Source: CAD feature listing. Evaluate the final solid. Frame: model axes, mm. Face numbers are marked on the shaded views. A direction names the side the tool comes from. Give positions to 0.01 mm unless a question says otherwise; leave off trailing zeros. Write each loop counter-clockwise with the first axis right and the second up, starting at its lowest first coordinate (ties: lowest second). Pieces come first, ordered by that corner, then holes. Notation, with made-up numbers: M 61.25,45 L 109.25,45 A20 ccw 109.25,71 Z; hole C 14,85.25 d7. An arc over 180 degrees is marked long. Use CSV: the item, a comma, the result in double quotes. Start each with the question number.
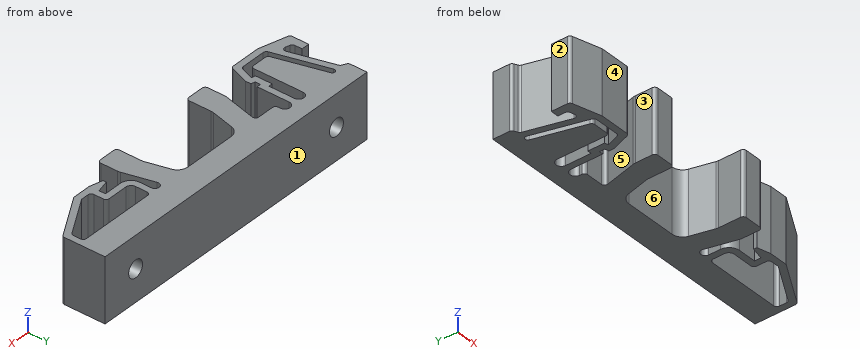
from build123d import *

# Parameters (mm, degrees)
BOSS_EXTRUDE1_DEPTH     = 6
CUT_EXTRUDE1_DEPTH      = 35.525353003
CUT_EXTRUDE1_DEPTH_BACK = 35.525353003
FILLET1_R               = 2
FILLET2_R               = 1
FILLET3_R               = 0.811424
FILLET4_R               = 2
FILLET5_R               = 1
FILLET6_R               = 1
FILLET7_R               = 0.5
FILLET8_R               = 0.6
SKETCH4_R               = 1.6
CUT_EXTRUDE2_DEPTH      = 8.5


with BuildPart() as part:
    # Sketch2 → Boss-Extrude1 (new, symmetric)
    with BuildSketch(Plane.XY):
        Polygon((6.5, 11), (-6.5, 11), (-8, 4.9838286), (-8, 0), (-12.25, 0), (-12.25, 3.981133366), (-10.5, 11), (-15, 11), (-15, 13), (-17, 13), (-17, 6), (-17.75, 6), (-17.75, 5), (-17, 4.813003998), (-17, 3.813003998), (-18.387819958, 0), (-24.387819958, 0), (-30, 1.50377911), (-30, 5.00377911), (-28.5, 5.00377911), (-28.5, 3.172407682), (-26.2783706, 2.577123878), (-28.785442178, 11.933642386), (-30, 12.5), (-30, 16), (0, 16), (30, 16), (30, 8), (21.339745962, 3), (17.839745962, 3), (15.4, 3.608296988), (15.4, 4.214079193), (17.75, 4.8), (17.75, 6), (12.35, 6), (12.35, 11), (10.5, 11), (12.25, 3.981133366), (12.25, 0), (8, 0), (8, 4.9838286), align=None)
    extrude(amount=BOSS_EXTRUDE1_DEPTH, both=True)

    # Sketch3 → Cut-Extrude1 (cut, two sides: drawn at the far end of the back side and taken through both)
    with BuildSketch(Plane.XY.offset(-CUT_EXTRUDE1_DEPTH_BACK)):
        Polygon((-27.626331186, 12.24422524), (-24.667039952, 1.2), (-19.228069004, 1.2), (-18.249764702, 3.88786898), (-18.95, 4.062457248), (-18.95, 7.2), (-18.2, 7.2), (-18.2, 13), (-20.2, 13), (-20.2, 2.2), (-23.899712964, 2.2), (-26.66040536, 12.503044285), align=None)
        Polygon((13.55, 11), (13.55, 7.2), (18.95, 7.2), (18.95, 4.2), (21.018206931, 4.2), (28.8, 8.692820323), (28.8, 11), align=None)
    extrude(amount=CUT_EXTRUDE1_DEPTH + CUT_EXTRUDE1_DEPTH_BACK, mode=Mode.SUBTRACT)

    # Fillet1
    fillet1_edges = [part.edges().sort_by_distance(p)[0] for p in [
        (12.35, 6, 0),
    ]]
    fillet(fillet1_edges, radius=FILLET1_R)

    # Fillet2
    fillet2_edges = [part.edges().sort_by_distance(p)[0] for p in [
        (13.55, 7.2, 0),
    ]]
    fillet(fillet2_edges, radius=FILLET2_R)

    # Fillet3
    fillet3_edges = [part.edges().sort_by_distance(p)[0] for p in [
        (12.35, 11, 0),
        (10.5, 11, 0),
    ]]
    fillet(fillet3_edges, radius=FILLET3_R)

    # Fillet4
    fillet4_edges = [part.edges().sort_by_distance(p)[0] for p in [
        (12.25, 3.981133366, 0),
        (8, 4.9838286, 0),
        (6.5, 11, 0),
        (-6.5, 11, 0),
        (-8, 4.9838286, 0),
        (-12.25, 3.981133366, 0),
    ]]
    fillet(fillet4_edges, radius=FILLET4_R)

    # Fillet5
    fillet5_edges = [part.edges().sort_by_distance(p)[0] for p in [
        (-20.2, 13, 0),
        (-18.2, 13, 0),
    ]]
    fillet(fillet5_edges, radius=FILLET5_R - 0.0001)  # a hair under: the kernel refuses the full size

    # Fillet6
    fillet6_edges = [part.edges().sort_by_distance(p)[0] for p in [
        (-15, 13, 0),
        (-17, 13, 0),
    ]]
    fillet(fillet6_edges, radius=FILLET6_R - 0.0001)  # a hair under: the kernel refuses the full size

    # Fillet7
    fillet7_edges = [part.edges().sort_by_distance(p)[0] for p in [
        (-27.626331186, 12.24422524, 0),
        (-26.66040536, 12.503044285, 0),
    ]]
    fillet(fillet7_edges, radius=FILLET7_R - 0.0001)  # a hair under: the kernel refuses the full size

    # Fillet8
    fillet8_edges = [part.edges().sort_by_distance(p)[0] for p in [
        (-23.899712964, 2.2, 0),
        (-20.2, 2.2, 0),
        (-19.228069004, 1.2, 0),
        (-24.667039952, 1.2, 0),
        (13.55, 11, 0),
        (28.8, 11, 0),
        (28.8, 8.692820323, 0),
        (18.95, 4.2, 0),
        (18.95, 7.2, 0),
        (12.25, 0, 0),
        (8, 0, 0),
        (-8, 0, 0),
        (-12.25, 0, 0),
        (-10.5, 11, 0),
        (-15, 11, 0),
        (-18.387819958, 0, 0),
        (-24.387819958, 0, 0),
        (-30, 1.50377911, 0),
        (-28.5, 3.172407682, 0),
        (-26.2783706, 2.577123878, 0),
        (-28.785442178, 11.933642386, 0),
        (-30, 12.5, 0),
        (30, 8, 0),
        (21.339745962, 3, 0),
        (17.839745962, 3, 0),
    ]]
    fillet(fillet8_edges, radius=FILLET8_R)

    # Sketch4 → Cut-Extrude2 (cut)
    with BuildSketch(Plane(origin=(0, 16, 0), x_dir=(1, 0, 0), z_dir=(0, 1, 0))):
        with Locations(Location((-23, 0, 0), (0, 0, 270))):
            Circle(SKETCH4_R)
        with Locations(Location((23, 0, 0), (0, 0, 180))):
            Circle(SKETCH4_R)
    extrude(amount=-CUT_EXTRUDE2_DEPTH, mode=Mode.SUBTRACT)


solid = part.part
Item 1: Contact query for flat-ended pins moving along their axis: pin 1 Ø3.5 at (x, z) = (19.5, -2.5) entering from -Y; pin 2 Ø0.7 at (y, z) = (9, -1) entering from -X; pin 3 Ø3.5 at (y, z) = (2.5, -2) entering from +X; pin 4 Ø1.5 at (x, y) = (-16, 2.5) entering from -Z. Output: stop coordinate, or through.
Item 2: Section A-A (y = 14). Return the cut outline in (x, z), plus the area to 3 significant figures.
Item 3: Section C-C (z = -2.25). State how many separate pieces and enclosed holes the cut face has, plus the area to 3 significant figures.
Item 4: Set-up query: the marked faces 4, 5 and 6. Return all of +Z, -Z, +X, -X, +Y, -Y with unobstructed straight access to the full face (end or side cutting, diameter ignored); none if empty.
Item 5: Material intervals for probe 1 along X at (y, z) = (12.5, 2); probe 2 along X at (y, z) = (1.5, 3); probe 3 along Z at (x, y) = (23, 12.8), sorted ascending.
Item 6: Section B-B (x = 23). Return the cut outline in (y, z).
Item 7: Pull-direction query (X, two-part tool) for the marked faces 1, 2 and 3; classes: released by +X, released by -X, zero draft, split by the parting line, or undercut.
Output values:
1,pin 1,"stops at y = 3"
1,pin 2,"stops at x = -28.09"
1,pin 3,"stops at x = 23.5"
1,pin 4,"passes through"
2,outline,"M -30,-6 L 30,-6 L 30,6 L -30,6 Z; hole C -23,0 d3.2; hole C 23,0 d3.2"
2,area,"704 mm2"
3,separate pieces,"1"
3,enclosed holes,"2"
3,area,"505 mm2"
4,face 4,"+Z, -Z, +X, -X, -Y"
4,face 5,"+Z, -Z"
4,face 6,"+Z, -Z, -Y"
5,probe 1,"x = -29.86 to -20.07, -18.33 to -16.87, -15.13 to 30"
5,probe 2,"x = -29.78 to -24.73, -19.13 to -17.84, -12.25 to -8, 8 to 12.25"
5,probe 3,"z = -6 to -1.6, 1.6 to 6"
6,outline,"M 3.96,-6 L 5.34,-6 L 5.34,6 L 3.96,6 Z; M 11,-6 L 16,-6 L 16,-1.6 L 11,-1.6 Z; M 11,1.6 L 16,1.6 L 16,6 L 11,6 Z"
7,face 1,"zero draft"
7,face 2,"released by -X"
7,face 3,"undercut"
